```python
from build123d import *

# Parameters (mm, degrees)
SKETCH1_R               = 5.55625
BOSS_EXTRUDE1_DEPTH     = 25.4
CUT_EXTRUDE1_DEPTH      = 44.994090512
CUT_EXTRUDE1_DEPTH_BACK = 44.994090512
SKETCH2_R               = 5.55625


with BuildPart() as part:
    # Sketch1 → Boss-Extrude1 (new body)
    with BuildSketch(Plane.XY):
        with BuildLine():
            ThreePointArc((-25.4, 0), (-21.680256121, -8.980256121), (-12.7, -12.7))
            Line((-12.7, -12.7), (25.4, -12.7))
            Line((25.4, -12.7), (25.4, 12.7))
            Line((25.4, 12.7), (-12.7, 12.7))
            ThreePointArc((-12.7, 12.7), (-21.680256121, 8.980256121), (-25.4, 0))
        make_face()
        with Locations((-12.7, 0)):
            Circle(SKETCH1_R, mode=Mode.SUBTRACT)
    extrude(amount=BOSS_EXTRUDE1_DEPTH)

    # Sketch2 → Cut-Extrude1 (cut, two sides: drawn at the far end of the back side and taken through both)
    with BuildSketch(Plane(origin=(0, 12.7, 0), x_dir=(1, 0, 0), z_dir=(0, 1, 0)).offset(-CUT_EXTRUDE1_DEPTH_BACK)):
        with Locations(Location((12.7, -12.7, 0), (0, 0, 270))):
            Circle(SKETCH2_R)
        with BuildLine():
            Line((25.4, 0), (12.7, 0))
            ThreePointArc((12.7, 0), (21.680256121, -3.719743879), (25.4, -12.7))
            Line((25.4, -12.7), (25.4, 0))
        make_face()
        with BuildLine():
            Line((25.4, -25.4), (25.4, -12.7))
            ThreePointArc((25.4, -12.7), (21.680256121, -21.680256121), (12.7, -25.4))
            Line((12.7, -25.4), (25.4, -25.4))
        make_face()
    extrude(amount=CUT_EXTRUDE1_DEPTH + CUT_EXTRUDE1_DEPTH_BACK, mode=Mode.SUBTRACT)


solid = part.part
```
Build history of the part. All positions in model axes, mm. Coordinates: 2 decimals unless noted, no trailing zeros. Order: outer loops, then holes, each group sorted by start corner. A loop starts at its lowest first (then second) coordinate and runs counter-clockwise, first axis right, second up. Notation, with made-up numbers: M -16,-23 L 39,-23 A24 cw 39,-7 Z; hole C -10,0 d1. An arc over 180 degrees is marked long. One line per question, with ' | ' between items. Start each with the question number.
1. Flat gauge pins, fed straight in: P1, Ø10, axis at x = 12.7, z = 12.7, coming from the -Y side; P2, Ø1, axis at x = 15, y = -5, coming from the +Z side; P3, Ø6, axis at x = 17, y = 9, coming from the -Z side; P4, Ø1.5, axis at y = -7.5, z = 5, coming from the +X side. Where does each tip first touch, or does it go through?
2. Cut at A-A (y = -2.75). Write the cut outline in (x, z).
3. Cut at C-C (x = -14). Write the cut outline in (y, z).
4. Wall check: line 1 along Y through (x, z) = (-12.7, 20.25); line 2 along Z through (x, y) = (12.7, -4.75); line 3 along X through (y, z) = (-1.25, 12.7). Give the ranges that are in metal, low to high. Write a range as [from, to].
5. Mould opens along X. For faces 1 (the face through (-6.6, 0.2, 0)), 2 (the face through (-16.795, 3.755, 12.522)) say: +X half, -X half, draft (parallel to the pull), parting line (faces both ways), or undercut.
6. Cut at D-D (y = 7). Write the cut outline in (x, z), plus the area to 3 significant figures.
7. Cut at B-B (z = 17). Write the cut outline in (x, y), plus the area to 3 significant figures.
The answers:
1) P1: passes through | P2: stops at z = 25.27 | P3: stops at z = 0.07 | P4: stops at x = 23.33
2) outline: M -25.1,0 L -17.53,0 L -17.53,25.4 L -25.1,25.4 Z; M -7.87,0 L 12.7,0 A12.7 ccw 12.7,25.4 L -7.87,25.4 Z; hole C 12.7,12.7 d11.11
3) outline: M -12.63,0 L -5.4,0 L -5.4,25.4 L -12.63,25.4 Z; M 5.4,0 L 12.63,0 L 12.63,25.4 L 5.4,25.4 Z
4) line 1: y = [-12.7, -5.56], [5.56, 12.7] | line 2: z = [0, 7.14], [18.26, 25.4] | line 3: x = [-25.34, -18.11], [-7.29, 7.14], [18.26, 25.4]
5) face 1: draft | face 2: undercut
6) outline: M -23.3,0 L 12.7,0 A12.7 ccw 12.7,25.4 L -23.3,25.4 Z; hole C 12.7,12.7 d11.11 | area: 1,070 mm2
7) outline: M -12.7,-12.7 L 9.18,-12.7 L 9.18,12.7 L -12.7,12.7 A12.7 ccw Z; M 16.22,-12.7 L 24.65,-12.7 L 24.65,12.7 L 16.22,12.7 Z; hole C -12.7,0 d11.11 | area: 926 mm2
